Read the model definition and answer for the solid it produces. Units are mm, in the model's axes. Give positions to 0.01 mm unless a question says otherwise; leave off trailing zeros. Order: outer loops, then holes, each group sorted by start corner. A loop starts at its lowest first (then second) coordinate and runs counter-clockwise, first axis right, second up. Notation, with made-up numbers: (80, -26) - (105, -26) arc R33 ccw to (105, 5) - close; hole circle Ø1 at (9.25, 47.25). An arc over 180 degrees is marked (long way). Use a Markdown table: item, result. Add a question column.
1. For a pull along Y with two mould halves and no side action, classify faces 1 (the flat face through (27, -13, 50.8)), 2 (the cylindrical face through (60.57, 19.07, 5.48)), 3 (the cylindrical face through (-1.21, -51.76, 25.76)) as released by +Y, released by -Y, zero draft, split by the parting line, or undercut.
2. Consider L1, parallel to Y at x = 0.5, z = 4; L2, parallel to Y at x = 0, z = 20.5; L3, parallel to X at y = 2, z = 3. Determine where each line is inside the solid, lowest interval first.
3. Flat-ended cylindrical pins translate along their axes: P1, Ø3, axis at x = 46.5, z = 17, coming from the +Y side; P2, Ø4, axis at y = -11, z = 5, coming from the +X side; P3, Ø5, axis at x = 8.5, z = 20.5, coming from the +Y side; P4, Ø6.5, axis at x = 0, y = 46.33, coming from the +Z side. Find the tip coordinate at first contact, or state that the pin passes through.
4. A cutting plane is placed at D-D on z = 44. Determine the outline of the cut face in (x, y).
5. A cutting plane is placed at C-C on z = 14.5. Determine the outline of the cut face in (x, y), and give its area (3 significant figures).
6. A cutting plane is placed at A-A on x = 0. Determine the outline of the cut face in (y, z), and give its area (3 significant figures).
```python
from build123d import *

# Parameters (mm, degrees)
F0_R     = 63.5
F0_R_2   = 28.1384603026
F1_DEPTH = 50.8
F2_R     = 11.0160883331
F4_R     = 5.5606419872
F5_DEPTH = 50.801


with BuildPart() as f1:
    # F0 (on Top) → F1 (new body)
    with BuildSketch(Plane.XY):
        Circle(F0_R)
        Circle(F0_R_2, mode=Mode.SUBTRACT)
    extrude(amount=F1_DEPTH)

    # F3: sweep along a path in F3_path
    with BuildLine(Plane(origin=(63.5, 0, 50.8), x_dir=(0, 1, 0), z_dir=(0, 0, 1))) as f3_path:
        CenterArc((0, 63.5), 63.5, 0, 360)
    # F2 (on Right) → F3 (sweep, cut)
    with BuildSketch(Plane.YZ):
        with Locations((63.3453205228, 22.1318639815)):
            Circle(F2_R)
    sweep(path=f3_path.line, mode=Mode.SUBTRACT)

    # F4 (on face) → F5 (cut, through all)
    with BuildSketch(Plane.XY.offset(50.8)):
        with Locations((0, -46.334028244)):
            Circle(F4_R)
        with Locations((46.334028244, 0)):
            Circle(F4_R)
        with Locations((0, 46.334028244)):
            Circle(F4_R)
        with Locations((-46.334028244, 0)):
            Circle(F4_R)
    extrude(amount=-F5_DEPTH, mode=Mode.SUBTRACT)


solid = f1.part
```
Output values:
| question | item | result |
|---|---|---|
| 1 | face 1 | zero draft |
| 1 | face 2 | split by the parting line |
| 1 | face 3 | undercut |
| 2 | L1 | -63.5 to -51.87, -40.8 to -28.13, 28.13 to 40.8, 51.87 to 63.5 |
| 2 | L2 | -52.45 to -51.89, -40.77 to -28.14, 28.14 to 40.77, 51.89 to 52.45 |
| 2 | L3 | -63.47 to -51.52, -41.15 to -28.07, 28.07 to 41.15, 51.52 to 63.47 |
| 3 | P1 | y = 29.63 |
| 3 | P2 | x = 62.86 |
| 3 | P3 | y = 52.52 |
| 3 | P4 | through |
| 4 | outline | circle Ø127 at (0, 0); hole circle Ø11.12 at (-46.33, 0); hole circle Ø56.28 at (0, 0); hole circle Ø11.12 at (0, -46.33); hole circle Ø11.12 at (0, 46.33); hole circle Ø11.12 at (46.33, 0) |
| 5 | outline | circle Ø110.8 at (0, 0); hole circle Ø11.12 at (-46.33, 0); hole circle Ø56.28 at (0, 0); hole circle Ø11.12 at (0, -46.33); hole circle Ø11.12 at (0, 46.33); hole circle Ø11.12 at (46.33, 0) |
| 5 | area | 6,770 mm² |
| 6 | outline | (-63.5, 0) - (-51.89, 0) - (-51.89, 50.8) - (-63.5, 50.8) - (-63.5, 33.15) arc R11.02 cw (long way) to (-63.5, 11.12) - close; (-40.77, 0) - (-28.14, 0) - (-28.14, 50.8) - (-40.77, 50.8) - close; (28.14, 0) - (40.77, 0) - (40.77, 50.8) - (28.14, 50.8) - close; (51.89, 0) - (63.5, 0) - (63.5, 11.12) arc R11.02 cw (long way) to (63.5, 33.15) - (63.5, 50.8) - (51.89, 50.8) - close |
| 6 | area | 2,070 mm² |
